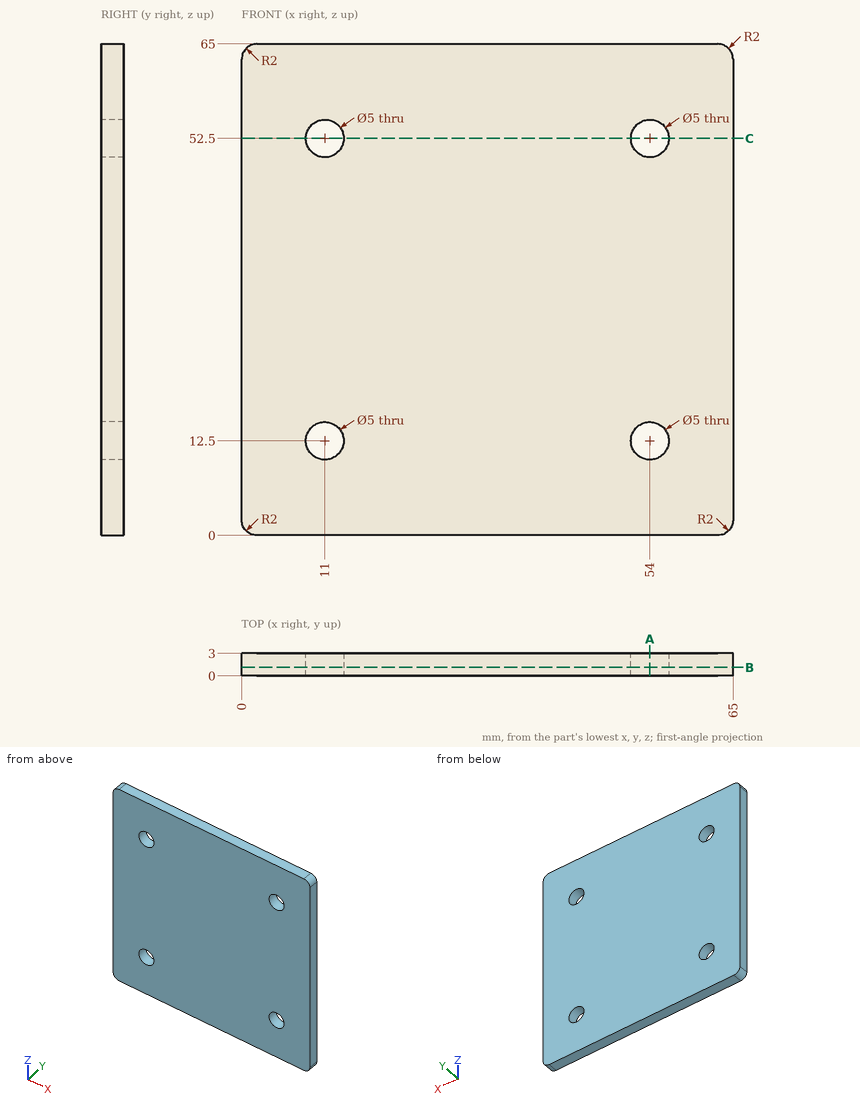
The drawing under review shows one solid part. Ordinate dimensions are in mm from its lowest x, y, z. Coordinates: 2 decimals unless noted, no trailing zeros. Order: outer loops, then holes, each group sorted by start corner. A loop starts at its lowest first (then second) coordinate and runs counter-clockwise, first axis right, second up. Notation, with made-up numbers: (-27, 45.5) -> (-7, 45.5) arc R27 cw to (-7, 74.5) -> close; hole circle Ø5 at (69, -27.75). An arc over 180 degrees is marked (long way). Use CSV: the item, a comma, the result in double quotes. Start each with the question number.
Item 1: We need section C-C, the plane z = 52.5. Give the boundary of the cut face in (x, y).
Item 2: Wall thickness on probe 1 along Z at (x, y) = (54, 0.8); probe 2 along Z at (x, y) = (54.5, 2.4): over which ranges is each line inside the solid? List them lowest first.
Item 3: We need section B-B, the plane y = 1.15. Give the boundary of the cut face in (x, z).
Item 4: Insertion check: pin 1 (4 mm diameter, centred on x = 11, z = 12.5, fed in from +Y). The pin has a flat end and moves straight along its axis. Give the tip position at first contact, or say it passes through.
Item 5: We need section A-A, the plane x = 54. Give the boundary of the cut face in (y, z), then the cut area to 3 significant figures.
Derived:
1,outline,"(0, 0) -> (8.5, 0) -> (8.5, 3) -> (0, 3) -> close; (13.5, 0) -> (51.5, 0) -> (51.5, 3) -> (13.5, 3) -> close; (56.5, 0) -> (65, 0) -> (65, 3) -> (56.5, 3) -> close"
2,probe 1,"z = 0 to 10, 15 to 50, 55 to 65"
2,probe 2,"z = 0 to 10.05, 14.95 to 50.05, 54.95 to 65"
3,outline,"(0, 2) arc R2 ccw to (2, 0) -> (63, 0) arc R2 ccw to (65, 2) -> (65, 63) arc R2 ccw to (63, 65) -> (2, 65) arc R2 ccw to (0, 63) -> close; hole circle Ø5 at (11, 12.5); hole circle Ø5 at (11, 52.5); hole circle Ø5 at (54, 12.5); hole circle Ø5 at (54, 52.5)"
4,pin 1,"passes through"
5,outline,"(0, 0) -> (3, 0) -> (3, 10) -> (0, 10) -> close; (0, 15) -> (3, 15) -> (3, 50) -> (0, 50) -> close; (0, 55) -> (3, 55) -> (3, 65) -> (0, 65) -> close"
5,area,"165 mm^2"
